Could you check a few things on this model? Use its own coordinates, in mm. A direction names the side the tool comes from. Round coordinates to 2 decimals unless told otherwise and drop trailing zeros. Write each loop counter-clockwise with the first axis right and the second up, starting at its lowest first coordinate (ties: lowest second). Pieces come first, ordered by that corner, then holes. Notation, with made-up numbers: (53.5, 49.5) - (91.5, 49.5) arc R11 cw to (91.5, 58.5) - close; hole circle Ø8 at (59.5, -8). An arc over 180 degrees is marked (long way). Put each result on its own line as item: value.
from build123d import *

# Parameters (mm, degrees)
F2_W     = 63.5
F2_H     = 63.5
F3_DEPTH = 9.526
F5_D     = 2.2606


with BuildPart() as f1:
    # F0 (on Right) → F1 (revolve)
    with BuildSketch(Plane.YZ):
        Polygon((0, 25.4), (0, 6.35), (3.6322, 6.35), (3.6322, 26.9875), (7.9248, 26.9875), (7.9248, 30.1625), (9.525, 30.1625), (9.525, 36.5125), (2.032, 36.5125), (2.032, 25.4), align=None)
    revolve(axis=Axis((0, 1.8161, 0), (0, -1, 0)))

    # F2 (on Front) → F3 (intersect, through all)
    with BuildSketch(Plane.XZ):
        Rectangle(F2_W, F2_H)
    extrude(amount=-F3_DEPTH, mode=Mode.INTERSECT)

    # F5 (through all)
    with Locations(Plane(origin=(0, 9.525, 0), x_dir=(-1, 0, 0), z_dir=(0, 1, 0))):
        with Locations((-22.4506403027, 22.4506403027), (22.4506403027, 22.4506403027), (22.4506403027, -22.4506403027), (-22.4506403027, -22.4506403027)):
            Hole(F5_D / 2)


solid = f1.part
(1) I'm going to push flat-ended pins straight in: pin 1 (2 mm diameter, centred on y = 5.5, z = 21.5, fed in from +X); pin 2 (5 mm diameter, centred on x = 20, z = 3, fed in from +Y); pin 3 (1.5 mm diameter, centred on x = 1, y = 1, fed in from -Z). Where does each tip first touch, or does it pass through?
Values found:
pin 1: stops at x = 30.21
pin 2: stops at y = 3.63
pin 3: stops at z = -25.4
(2) If we mould it in two halves opening along X, with no side actions, what happens to faces 4 (the face through (24.796, 1.002, -5.506)), 5 (the face through (-31.75, 6, 0)), 6 (the face through (15.5, 7.925, 22.5))? For each: pulls with the +X half, pulls with the -X half, needs draft (parallel to the pull), parting line crosses it, or undercut.
Values found:
face 4: parting line crosses it
face 5: pulls with the -X half
face 6: undercut
(3) Imagine slicing it at C-C, the plane x = -10.5. List the corners of the cut face in (y, z) for me (3 decimals).
Values found:
outline: (0, -23.128) - (2.032, -23.128) - (2.032, -31.75) - (9.525, -31.75) - (9.525, -28.276) - (7.925, -28.276) - (7.925, -24.861) - (3.632, -24.861) - (3.632, 24.861) - (7.925, 24.861) - (7.925, 28.276) - (9.525, 28.276) - (9.525, 31.75) - (2.032, 31.75) - (2.032, 23.128) - (0, 23.128) - close
(4) Please list where these lines run through material, in increasing order: probe 1 along X at (y, z) = (4.55, 0); probe 2 along X at (y, z) = (9, 0); probe 3 along X at (y, z) = (8.5, -23). Write a range as from..to.
Values found:
probe 1: x = -31.75..-26.99, 26.99..31.75
probe 2: x = -31.75..-30.16, 30.16..31.75
probe 3: x = -28.36..-23.44, -21.46..-19.51, 19.51..21.46, 23.44..28.36
(5) For faces 1 (the face through (-22, 2.032, -15)), 2 (the face through (-1.326, 8.736, -30.133)), 3 (the face through (22.972, 5.726, -23.453)), which set-ups out of +Z, -Z, +X, -X, +Y, -Y let a thin tool reach every point of the face, with its end or its side?
Values found:
face 1: -Y
face 2: +Y
face 3: +Y, -Y
